Part model, mm, in its own coordinate system. Give positions to 0.01 mm unless a question says otherwise; leave off trailing zeros. Write each loop counter-clockwise with the first axis right and the second up, starting at its lowest first coordinate (ties: lowest second). Pieces come first, ordered by that corner, then holes. Notation, with made-up numbers: M 48,-26 L 93,-26 A23 ccw 93,2 Z; hole C 62,-24.5 d10. An arc over 180 degrees is marked long. Answer as CSV lines item,"result". Start each with the question number.
1) Slice it at D-D, the plane x = -9. Give the cut face in (y, z).
2) Mould opens along X. For faces 1 (the flat face through (0, 14.759, 1)), 2 (the cylindrical face through (-17.258, 7.734, 0.76)), 3 (the cylindrical face through (-12.76, 11.742, 0.74)), 4 (the cylindrical face through (6.33, -9.46, 0.74)) say: pulls with the +X half, pulls with the -X half, needs draft (parallel to the pull), parting line crosses it, or undercut.
3) Slice it at B-B, the plane y = -7.25. Give the cut face in (x, z), plus the area to 3 significant figures.
4) Slice it at A-A, the plane x = 6.5. Give the cut face in (y, z).
5) Slice it at C-C, the plane z = 0.7. Give the cut face in (x, y).
6) Wall check: line 1 along X through (y, z) = (10.5, 1.3); line 2 along X through (y, z) = (8, 0.3); line 3 along Y through (x, z) = (-12.5, 0.65). Give the ranges that are in metal, low to high. Write a range as from..to.
```python
from build123d import *

# Parameters (mm, degrees)
SKETCH_1_R      = 2
EXTRUDE_1_DEPTH = 1.5
FILLET_1_R      = 3


with BuildPart() as part:
    # ｽｹｯﾁ1 → ﾎﾞｽ - 押し出し1 (new body)
    with BuildSketch(Plane.XY):
        Polygon((-17.5, 7.650184139), (5.495827016, -14.759182375), (17.5, -2.440856231), (17.5, 14.759182375), (-17.5, 14.759182375), align=None)
        with Locations((5.404503628, -7.688704312)):
            Circle(SKETCH_1_R, mode=Mode.SUBTRACT)
        with Locations((-12.5, 9.759182375)):
            Circle(SKETCH_1_R, mode=Mode.SUBTRACT)
        with Locations((12.5, 9.759182375)):
            Circle(SKETCH_1_R, mode=Mode.SUBTRACT)
    extrude(amount=EXTRUDE_1_DEPTH)

    # ﾌｨﾚｯﾄ1
    fillet_1_edges = [part.edges().sort_by_distance(p)[0] for p in [
        (-17.5, 7.650184139, 0.75),
        (-17.5, 14.759182375, 0.75),
        (17.5, 14.759182375, 0.75),
        (17.5, -2.440856231, 0.75),
        (5.495827016, -14.759182375, 0.75),
    ]]
    fillet(fillet_1_edges, radius=FILLET_1_R)


solid = part.part
```
Found:
1,outline,"M -0.63,0 L 14.76,0 L 14.76,1.5 L -0.63,1.5 Z"
2,face 1,"needs draft"
2,face 2,"pulls with the -X half"
2,face 3,"undercut"
2,face 4,"undercut"
3,outline,"M -2.21,0 L 3.45,0 L 3.45,1.5 L -2.21,1.5 Z; M 7.36,0 L 12.81,0 L 12.81,1.5 L 7.36,1.5 Z"
3,area,"16.7 mm²"
4,outline,"M -13.32,0 L -9.36,0 L -9.36,1.5 L -13.32,1.5 Z; M -6.02,0 L 14.76,0 L 14.76,1.5 L -6.02,1.5 Z"
5,outline,"M -17.5,8.92 A3 ccw -16.59,6.77 L 3.35,-12.67 A3 ccw 7.59,-12.61 L 16.65,-3.31 A3 ccw 17.5,-1.22 L 17.5,11.76 A3 ccw 14.5,14.76 L -14.5,14.76 A3 ccw -17.5,11.76 Z; hole C -12.5,9.76 d4; hole C 5.4,-7.69 d4; hole C 12.5,9.76 d4"
6,line 1,"-17.5..-14.36, -10.64..10.64, 14.36..17.5"
6,line 2,"-17.36..-13.45, -11.55..11.55, 13.45..17.5"
6,line 3,"2.78..7.76, 11.76..14.76"
